Can you work these out from the model? Positions are in its coordinate system, mm. Face numbers are marked on the shaded views. A direction names the side the tool comes from. Round coordinates to 2 decimals unless told otherwise and drop trailing zeros. Write each loop counter-clockwise with the first axis right and the second up, starting at its lowest first coordinate (ties: lowest second). Pieces come first, ordered by that corner, then holes. Notation, with made-up numbers: M -12.75,38.5 L -7.75,38.5 A20 cw -7.75,43.5 Z; hole C 55.25,71.25 d2. An arc over 180 degrees is marked long. Answer as a JSON object with one key per item and string values. Group by question number.
1) Suppose I cut it at D-D, the plane z = -5. Write out the boundary of the cut face in (x, y).
2) Please list where these lines run through material, in increasing order: L1, parallel to X at y = 3.25, z = 4; L2, parallel to Y at x = -1.75, z = 2.25; L3, parallel to X at y = 0.75, z = -6. Write a range as [from, to].
3) Suppose I cut it at C-C, the plane z = 2.5. Write out the boundary of the cut face in (x, y), and give its area (3 significant figures).
4) I'm going to push flat-ended pins straight in: pin 1 Ø3.5 at (x, z) = (5.43, 5) entering from +Y; pin 2 Ø1.6 at (y, z) = (5, 2.5) entering from +X. Where does each tip first touch, or does it pass through?
5) Suppose I cut it at A-A, the plane z = 0. Write out the boundary of the cut face in (x, y), and give its area (3 significant figures).
6) If we mould it in two halves opening along X, with no side actions, what happens to the marked faces 1, 2, 3 and 4? For each: +X half, -X half, draft (parallel to the pull), parting line (faces both ways), or undercut.
7) Suppose I cut it at B-B, the plane y = 5.5. Write out the boundary of the cut face in (x, z).
8) On a 3-axis mill with a long thin cutter (end or side, diameter ignored), from which of +Z, -Z, +X, -X, +Y, -Y can I reach the whole of each face in a straight line? I mean the marked faces 5 and 6. Say none if no direction works.
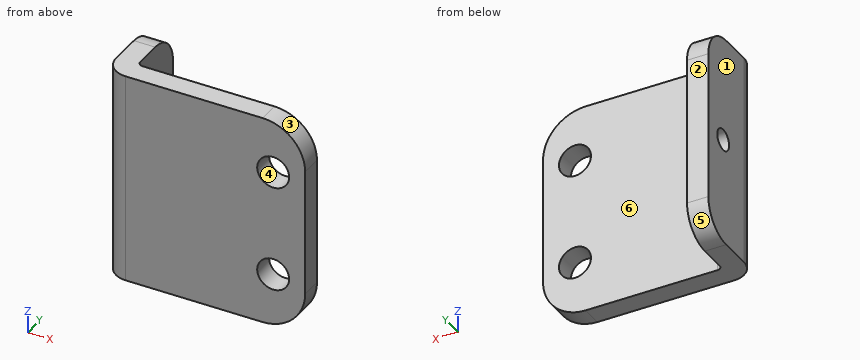
from build123d import *

# Parameters (mm, degrees)
SKETCH1_W           = 16.852791878
SKETCH1_H           = 20
BOSS_EXTRUDE1_DEPTH = 2
FILLET1_R           = 4
SKETCH2_W           = 20
SKETCH2_H           = 8
SKETCH2_R           = 1
BOSS_EXTRUDE2_DEPTH = 2
FILLET2_R           = 3
FILLET3_R           = 3
FILLET4_R           = 2
FILLET5_R           = 0.5
SKETCH3_R           = 1.5
CUT_EXTRUDE1_DEPTH  = 16.643200832


with BuildPart() as part:
    # Sketch1 → Boss-Extrude1 (new body)
    with BuildSketch(Plane(origin=(0, 0, 0), x_dir=(1, 0, 0), z_dir=(0, 1, 0))):
        Rectangle(SKETCH1_W, SKETCH1_H)
    extrude(amount=BOSS_EXTRUDE1_DEPTH)

    # Fillet1
    fillet1_edges = [part.edges().sort_by_distance(p)[0] for p in [
        (8.426395939, 1, 10),
        (8.426395939, 1, -10),
    ]]
    fillet(fillet1_edges, radius=FILLET1_R)

    # Sketch2 → Boss-Extrude2 (add)
    with BuildSketch(Plane.ZY.offset(8.426395939)):
        with Locations((0, 4)):
            Rectangle(SKETCH2_W, SKETCH2_H)
        with Locations((0, 5.5)):
            Circle(SKETCH2_R, mode=Mode.SUBTRACT)
    extrude(amount=BOSS_EXTRUDE2_DEPTH)

    # Fillet2
    fillet2_edges = [part.edges().sort_by_distance(p)[0] for p in [
        (-9.426395939, 8, 10),
    ]]
    fillet(fillet2_edges, radius=FILLET2_R)

    # Fillet3
    fillet3_edges = [part.edges().sort_by_distance(p)[0] for p in [
        (-9.426395939, 8, -10),
    ]]
    fillet(fillet3_edges, radius=FILLET3_R)

    # Fillet4
    fillet4_edges = [part.edges().sort_by_distance(p)[0] for p in [
        (-10.426395939, 0, 0),
    ]]
    fillet(fillet4_edges, radius=FILLET4_R)

    # Fillet5
    fillet5_edges = [part.edges().sort_by_distance(p)[0] for p in [
        (-8.426395939, 2, 0),
    ]]
    fillet(fillet5_edges, radius=FILLET5_R)

    # Sketch3 → Cut-Extrude1 (cut, through all)
    with BuildSketch(Plane(origin=(0, 2, 0), x_dir=(1, 0, 0), z_dir=(0, 1, 0))):
        with Locations(Location((5.426395939, 5, 0), (0, 0, 270))):
            Circle(SKETCH3_R)
        with Locations(Location((5.426395939, -5, 0), (0, 0, 270))):
            Circle(SKETCH3_R)
    extrude(amount=-CUT_EXTRUDE1_DEPTH, mode=Mode.SUBTRACT)


solid = part.part
Results:
{
 "1": {"outline": "M -10.43,2 A2 ccw -8.43,0 L 3.93,0 L 3.93,2 L -7.93,2 A0.5 cw -8.43,2.5 L -8.43,8 L -10.43,8 Z; M 6.93,0 L 8.43,0 L 8.43,2 L 6.93,2 Z"},
 "2": {"L1": "[-10.43, -8.43]", "L2": "[0, 2]", "L3": "[-9.99, 4.31], [6.54, 8.43]"},
 "3": {"outline": "M -10.43,2 A2 ccw -8.43,0 L 8.43,0 L 8.43,2 L -7.93,2 A0.5 cw -8.43,2.5 L -8.43,8 L -10.43,8 Z", "area": "48.9 mm^2"},
 "4": {"pin 1": "y = 2", "pin 2": "x = -8.43"},
 "5": {"outline": "M -10.43,2 A2 ccw -8.43,0 L 8.43,0 L 8.43,2 L -7.93,2 A0.5 cw -8.43,2.5 L -8.43,4.5 L -10.43,4.5 Z; M -10.43,6.5 L -8.43,6.5 L -8.43,8 L -10.43,8 Z", "area": "44.9 mm^2"},
 "6": {"face 1": "-X half", "face 2": "draft", "face 3": "+X half", "face 4": "undercut"},
 "7": {"outline": "M -10.43,-9.96 L -8.43,-9.96 L -8.43,-1 L -10.43,-1 Z; M -10.43,1 L -8.43,1 L -8.43,9.96 L -10.43,9.96 Z"},
 "8": {"face 5": "-Z, +X, -X, +Y", "face 6": "+Z, -Z, +X, +Y"}
}
